```python
from build123d import *

# Parameters (mm, degrees)
F1_DEPTH  = 75
F2_W      = 150
F2_H      = 75
F3_DEPTH  = 1500
F4_W      = 70
F4_H      = 200
F5_DEPTH  = 75.001
F6_W      = 6
F6_H      = 20
F7_DEPTH  = 40
F8_R      = 9.99999
F9_R      = 3.25
F10_DEPTH = 507.501
F12_R     = 12.5
F13_DEPTH = 575.001


# Not quite as in the source:
# - a fillet or chamfer is up to 0.001 mm smaller than in the source, because OpenCascade refuses the exact size
# - a feature of the source that left no trace in its solid (it failed there, or was rolled back) is left out


with BuildPart() as f1:
    # F0 (on Top) → F1 (new body)
    with BuildSketch(Plane.XY):
        Polygon((500, 0), (-500, 0), (-500, -1000), (-425, -1000), (-425, -75), (425, -75), (425, -1000), (500, -1000), align=None)
    extrude(amount=F1_DEPTH)

    # F2 (on face) → F3 (join)
    with BuildSketch(Plane.XY.offset(75)):
        with Locations((0, -37.5)):
            Rectangle(F2_W, F2_H)
    extrude(amount=F3_DEPTH)

    # F4 (on face) → F5 (cut, through all)
    with BuildSketch(Plane.XZ.offset(75)):
        with Locations((0, 1425)):
            Rectangle(F4_W, F4_H)
    extrude(amount=-F5_DEPTH, mode=Mode.SUBTRACT)

    # F6 (on face) → F7 (join)
    with BuildSketch(Plane(origin=(0, 0, 0), x_dir=(-1, 0, 0), z_dir=(0, 1, 0))):
        with Locations((-4.5, 710)):
            Rectangle(F6_W, F6_H)
        with Locations((10.5, 710)):
            Rectangle(F6_W, F6_H)
    extrude(amount=F7_DEPTH)

    # F8 (radius 10 in the source; OpenCascade refuses exactly that, so slightly less here)
    f8_edges = [f1.edges().sort_by_distance(p)[0] for p in [
        (4.5, 40, 720),
        (4.5, 40, 700),
        (-10.5, 40, 720),
        (-10.5, 40, 700),
    ]]
    fillet(f8_edges, radius=F8_R)

    # F9 (on face) → F10 (cut, through all)
    with BuildSketch(Plane.YZ.offset(7.5)):
        with Locations((31, 710)):
            Circle(F9_R)
    extrude(amount=-F10_DEPTH, mode=Mode.SUBTRACT)

    # F12 (on face) → F13 (cut, through all)
    with BuildSketch(Plane(origin=(-75, 0, 0), x_dir=(0, -1, 0), z_dir=(-1, 0, 0))):
        with Locations((37.5, 1425)):
            Circle(F12_R)
    extrude(amount=-F13_DEPTH, mode=Mode.SUBTRACT)


solid = f1.part
```
Design review of the part built by this model. Coordinates are the model's own, in mm. A direction names the side the tool comes from. Give positions to 0.01 mm unless a question says otherwise; leave off trailing zeros. Loops run counter-clockwise (first coordinate to the right, second up) from the corner with the lowest first, then second, coordinate; pieces in that order, holes last. Notation, with made-up numbers: (80, -13.5) -> (94, -13.5) arc R10 cw to (94, -6.5) -> close; hole circle Ø11 at (46, 30). An arc over 180 degrees is marked (long way). Write each question's results on one line, items separated by ' | '.
Q1. Take a section at A-A, the plane y = -500. Write out the cut boundary in (x, z).
Reply:
outline: (-500, 0) -> (-425, 0) -> (-425, 75) -> (-500, 75) -> close; (425, 0) -> (500, 0) -> (500, 75) -> (425, 75) -> close
Q2. Take a section at B-B, the plane x = -265.5. Write out the cut boundary in (y, z), plus the area to 4 significant figures.
Reply:
outline: (-75, 0) -> (0, 0) -> (0, 75) -> (-75, 75) -> close | area: 5,625 mm²
Q3. Take a section at C-C, the plane z = 1091. Write out the cut boundary in (x, y), plus the area to 4 significant figures.
Reply:
outline: (-75, -75) -> (75, -75) -> (75, 0) -> (-75, 0) -> close | area: 11,250 mm²
Q4. For pin 1 Ø16 at (y, z) = (22, 708) entering from -X; pin 2 Ø22 at (y, z) = (12, 714.5) entering from +X; pin 3 Ø22.5 at (y, z) = (-56, 934) entering from -X; pin 4 Ø6 at (y, z) = (31, 710) entering from -X, all flat-tipped, find the tip position at first contact; note any pin that passes through.
Reply:
pin 1: stops at x = -13.5 | pin 2: stops at x = 7.5 | pin 3: stops at x = -75 | pin 4: passes through
Q5. Wall thickness on L1, parallel to Z at x = -11.35, y = 31; L2, parallel to Z at x = 59.5, y = -37.5; L3, parallel to Y at x = 60, z = 1425: over which ranges is each line inside the solid? List them lowest first.
Reply:
L1: z = 700.05 to 706.75, 713.25 to 719.95 | L2: z = 0 to 1412.5, 1437.5 to 1575 | L3: y = -75 to -50, -25 to 0
Q6. Machinability: for faces 1 (the face through (-1, -37, 1575)), 2 (the face through (-75, -38, 814)), 3 (the face through (0, -38, 1525)), 4 (the face through (75, -38, 814)), 5 (the face through (425, -531, 37)), which of the approach directions +Z, -Z, +X, -X, +Y, -Y give a long, thin tool a straight path to every point of the face, cutting with its end or side? Answer none if there is none.
Reply:
face 1: +Z, +X, -X, +Y, -Y | face 2: +Z, -X, +Y, -Y | face 3: +Y, -Y | face 4: +Z, +X, +Y, -Y | face 5: +Z, -Z, -Y
